For this review, take the finished solid that the model builds, in its own axes (mm). Face numbers are marked on the shaded views. A direction names the side the tool comes from. Coordinates: 2 decimals unless noted, no trailing zeros. Write each loop counter-clockwise with the first axis right and the second up, starting at its lowest first coordinate (ties: lowest second). Pieces come first, ordered by that corner, then holes. Notation, with made-up numbers: (51.5, 76) -> (83.5, 76) arc R24 ccw to (83.5, 97) -> close; hole circle Ø8 at (-37, 61.5). An arc over 180 degrees is marked (long way). Put each result on its own line as item: value. Start each with the question number.
Item 1: Consider section B-B on x = -115. Give the boundary of the cut face in (y, z).
Item 2: The part is to be moulded in two halves that separate along Y. For the marked faces 1, 2 and 3, say which applies: +Y half, -Y half, draft (parallel to the pull), parting line (faces both ways), or undercut.
Item 3: For the marked faces 4, 5 and 6, list the 3-axis set-ups (+Z, -Z, +X, -X, +Y, -Y) from which the entire face can be reached by the end or side of a thin tool; tool diameter is ignored.
Item 4: Consider section A-A on y = 13. Give the boundary of the cut face in (x, z).
Item 5: Insertion check: P1, Ø5, axis at y = 124.5, z = 17.5, coming from the +X side; P2, Ø12, axis at y = 206, z = 25, coming from the -X side; P3, Ø1, axis at y = 151.5, z = 21.5, coming from the -X side. Each pin has a flat end and moves straight along its axis. Give the tip position at first contact, or say it passes through.
Item 6: To check wall thickness, follow L1, parallel to Y at x = -86.5, z = 16.5; L2, parallel to Y at x = -90, z = 23; L3, parallel to X at y = 203.5, z = 18. State the ranges of each line that lie inside material, in increasing order.
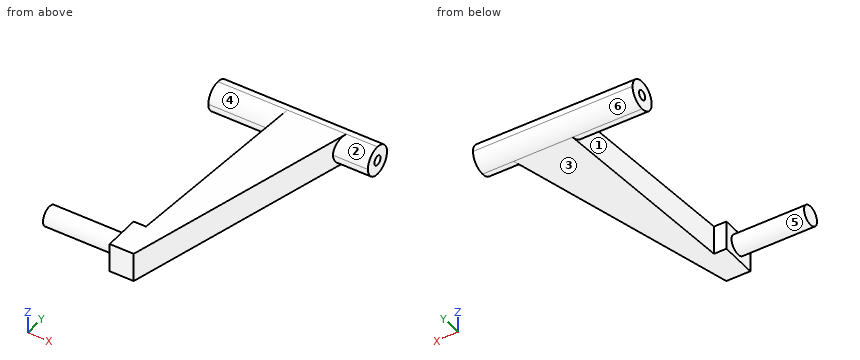
```python
from build123d import *

# Parameters (mm, degrees)
F1_DEPTH = 40
F2_R     = 19.99999
F3_R     = 6.5
F4_DEPTH = 220.001
F5_R     = 13.52259159
F6_DEPTH = 100


# Not quite as in the source:
# - a fillet or chamfer is up to 0.001 mm smaller than in the source, because OpenCascade refuses the exact size


with BuildPart() as f1:
    # F0 (on Top) → F1 (new body)
    with BuildSketch(Plane.XY):
        Polygon((125.4761886686, 235.2380912917), (-94.5238113314, 235.2380912917), (-94.5238113314, 195.2380912917), (0, 195.2380912917), (-15.9523813939, -54.7619087083), (-33.0952398201, -54.7619087083), (-33.0952398201, -104.7619087083), (0, -104.7619087083), (77.3809560928, 195.2380912917), (125.4761886686, 195.2380912917), align=None)
    extrude(amount=F1_DEPTH)

    # F2 (radius 20 in the source; OpenCascade refuses exactly that, so slightly less here)
    f2_edges = [f1.edges().sort_by_distance(p)[0] for p in [
        (15.476189, 235.238091, 40),
        (15.476189, 235.238091, 0),
        (-47.261906, 195.238091, 0),
        (-47.261906, 195.238091, 40),
        (101.428572, 195.238091, 0),
        (101.428572, 195.238091, 40),
    ]]
    fillet(f2_edges, radius=F2_R)

    # F3 (on face) → F4 (cut, through all)
    with BuildSketch(Plane(origin=(-94.5238113314, 0, 0), x_dir=(0, -1, 0), z_dir=(-1, 0, 0))):
        with Locations((-215.2380912917, 20)):
            Circle(F3_R)
    extrude(amount=-F4_DEPTH, mode=Mode.SUBTRACT)

    # F5 (on face) → F6 (join)
    with BuildSketch(Plane(origin=(-33.0952398201, 0, 0), x_dir=(0, -1, 0), z_dir=(-1, 0, 0))):
        with Locations((78.9996907115, 21.1079698056)):
            Circle(F5_R)
    extrude(amount=F6_DEPTH)


solid = f1.part
```
Return value:
1. outline: circle Ø27.05 at (-79, 21.11)
2. face 1: undercut
2. face 2: -Y half
2. face 3: draft
3. face 4: +Z, -X
3. face 5: -X
3. face 6: -Z, +X, -X, +Y
4. outline: (-11.63, 0) -> (30.38, 0) -> (30.38, 40) -> (-11.63, 40) -> close
5. P1: x = 59.78
5. P2: x = -94.52
5. P3: x = -2.82
6. L1: -91.71 to -66.29, 195.55 to 209.76, 220.72 to 234.93
6. L2: -92.39 to -65.61, 195.46 to 209.47, 221 to 235.01
6. L3: -94.52 to 125.48
